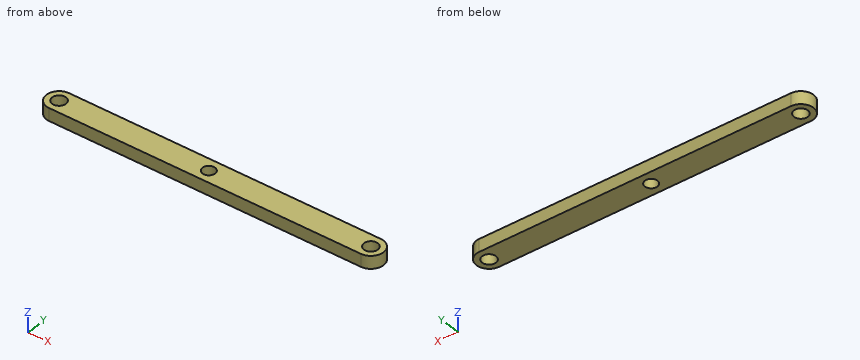
Autodesk Fusion 360 part; units mm, degrees
sketch "Boceto1" plane through (0, 0, 0) normal (0, 0, 1) x (1, 0, 0)
  line L0 (0, -23.8223) -> (0, 23.8223) construction
  circle A0 centre (64.256, 0) radius 2.75
  line L1 (-59.344, 5) -> (64.256, 5)
  line L2 (0, 0) -> (11, 0) construction
  line L3 (-59.344, -5) -> (64.256, -5)
  arc A1 (64.256, -5) -> (64.256, 5) centre (64.256, 0) ccw
  circle A2 centre (-59.344, 0) radius 2.75
  arc A3 (-59.344, 5) -> (-59.344, -5) centre (-59.344, 0) ccw
  dimension "d1" = 5.5
  dimension "d2" = 64.256
  dimension "d4" = 10
  dimension "d10" = 5.5
  dimension "d11" = 123.6
  dimension "d12" = 5
extrude "Extruir1" add sketch "Boceto1" along normal blind 5
sketch "Boceto2" plane through (0, 0, 5) normal (0, 0, 1) x (1, 0, 0)
  circle A0 centre (64.256, 0) radius 2.75
  line L0 (-59.344, -5) -> (64.256, -5)
  arc A1 (64.256, -5) -> (64.256, 5) centre (64.256, 0) ccw
  line L1 (64.256, 5) -> (-59.344, 5)
  circle A2 centre (0, 0) radius 2.5
  arc A3 (-59.344, 5) -> (-59.344, -5) centre (-59.344, 0) ccw
  circle A4 centre (-59.344, 0) radius 2.75
  dimension "d8" = 5
extrude "Extruir2" cut sketch "Boceto2" against normal through all contours A2
equation "d2 = ( 128.512 / 2 ) * 1 mm"
Here's how the part is built. I have some questions about the finished solid (model axes, mm). Round coordinates to 2 decimals unless told otherwise and drop trailing zeros. Loops run counter-clockwise (first coordinate to the right, second up) from the corner with the lowest first, then second, coordinate; pieces in that order, holes last. Notation, with made-up numbers: (70.5, -37) -> (91.5, -37) arc R18 ccw to (91.5, -6) -> close; hole circle Ø9 at (-7.75, 22). An arc over 180 degrees is marked (long way). Write each question's results on one line, items separated by ' | '.
(1) If we section it at A-A, the plane y = 0: List the corners of the cut face in (x, z) for me, then the cut area to 3 significant figures.
Worked answers:
outline: (-64.34, 0) -> (-62.09, 0) -> (-62.09, 5) -> (-64.34, 5) -> close; (-56.59, 0) -> (-2.5, 0) -> (-2.5, 5) -> (-56.59, 5) -> close; (2.5, 0) -> (61.51, 0) -> (61.51, 5) -> (2.5, 5) -> close; (67.01, 0) -> (69.26, 0) -> (69.26, 5) -> (67.01, 5) -> close | area: 588 mm2
(2) If we section it at C-C, the plane z = 4.25: List the corners of the cut face in (x, y) for me.
Worked answers:
outline: (-59.34, -5) -> (64.26, -5) arc R5 ccw to (64.26, 5) -> (-59.34, 5) arc R5 ccw to start; hole circle Ø5.5 at (-59.34, 0); hole circle Ø5 at (0, 0); hole circle Ø5.5 at (64.26, 0)
(3) If we section it at B-B, the plane x = 0: List the corners of the cut face in (y, z) for me.
Worked answers:
outline: (-5, 0) -> (-2.5, 0) -> (-2.5, 5) -> (-5, 5) -> close; (2.5, 0) -> (5, 0) -> (5, 5) -> (2.5, 5) -> close
(4) If I drill on L1, parallel to X at y = -0.25, z = 2.8; L2, parallel to X at y = 0.75, z = 0.5; L3, parallel to Y at x = 0, z = 2.75, over which ranges is the centre line in solid material (lowest first)?
Worked answers:
L1: -64.34 to -62.08, -56.61 to -2.49, 2.49 to 61.52, 66.99 to 69.25 | L2: -64.29 to -61.99, -56.7 to -2.38, 2.38 to 61.61, 66.9 to 69.2 | L3: -5 to -2.5, 2.5 to 5
